from build123d import *

# Parameters (mm, degrees)
SKETCH1_R               = 3.3147
BOSS_EXTRUDE1_DEPTH     = 22.225
SHELL1_START            = -19.05
SHELL1_OUTLINE_R        = 3.3147
SHELL1_DEPTH            = 38.1
F_1_2_CLEARANCE_HOLE1_D = 13.49248


# Read off the part's stored shape, not the designer's step: Shell1
with BuildPart() as part:
    # Sketch1 → Boss-Extrude1 (new, symmetric)
    with BuildSketch(Plane.XY):
        Polygon((41.275, -44.45), (1101.725, -44.45), (1101.725, 0), (0, 0), (0, -3.175), align=None)
        with Locations((1076.325, -22.225)):
            Circle(SKETCH1_R, mode=Mode.SUBTRACT)
    extrude(amount=BOSS_EXTRUDE1_DEPTH, both=True)

    # Shell1 outline → Shell1 (cut)
    with BuildSketch(Plane.XY.offset(SHELL1_START)):
        Polygon((38.1, -41.275), (1101.725, -41.275), (1101.725, -3.175), (0, -3.175), align=None)
        with Locations((1076.325, -22.225)):
            Circle(SHELL1_OUTLINE_R, mode=Mode.SUBTRACT)
    extrude(amount=SHELL1_DEPTH, mode=Mode.SUBTRACT)

    # 1/2 Clearance Hole1 (through all)
    with Locations(Plane(origin=(0, 0, 0), x_dir=(1, 0, 0), z_dir=(0, 1, 0))):
        with Locations((19.05, 0)):
            Hole(F_1_2_CLEARANCE_HOLE1_D / 2)


solid = part.part
Here's how the part is built. I have some questions about the finished solid (model axes, mm). A direction names the side the tool comes from. Round coordinates to 2 decimals unless told otherwise and drop trailing zeros. Order: outer loops, then holes, each group sorted by start corner. A loop starts at its lowest first (then second) coordinate and runs counter-clockwise, first axis right, second up. Notation, with made-up numbers: M 22.5,-9.5 L 44.5,-9.5 A28 ccw 44.5,14.5 Z; hole C 36,-18 d3. An arc over 180 degrees is marked long. One line per question, with ' | ' between items.
1) Imagine slicing it at C-C, the plane y = -11.5. Write out the boundary of the cut face in (x, z) (3 decimals).
Checked values:
outline: M 8.325,-22.225 L 1101.725,-22.225 L 1101.725,-19.05 L 8.325,-19.05 Z; M 8.325,19.05 L 1101.725,19.05 L 1101.725,22.225 L 8.325,22.225 Z
2) On a 3-axis mill with a long thin cutter (end or side, diameter ignored), from which of +Z, -Z, +X, -X, +Y, -Y can I reach the whole of each face in a straight line? I mean faces 5 (the flat face through (562, -41.275, 0)), 6 (the flat face through (543, -22, -22.225)). Say none if no direction works.
Checked values:
face 5: +X, -X | face 6: -Z, +X, -X, +Y, -Y
3) Imagine slicing it at A-A, the plane x = 894.5. Write out the boundary of the cut face in (y, z) (3 decimals).
Checked values:
outline: M -44.45,-22.225 L 0,-22.225 L 0,22.225 L -44.45,22.225 Z; hole M -41.275,-19.05 L -3.175,-19.05 L -3.175,19.05 L -41.275,19.05 Z
4) I need wall thicknesses on line 1 (Z direction, x = 740.5, y = -11.5) (3 decimals); line 2 (Y direction, x = 676, z = -10) (3 decimals); line 3 (Z direction, x = 19, y = -1) (3 decimals). Which ranges of each line are inside material? Lowest first, please.
Checked values:
line 1: z = -22.225 to -19.05, 19.05 to 22.225 | line 2: y = -44.45 to -41.275, -3.175 to 0 | line 3: z = -22.225 to -6.746, 6.746 to 22.225
5) Imagine slicing it at B-B, the plane z = 0. Write out the boundary of the cut face in (x, y) (3 decimals), plus the area to 3 significant figures.
Checked values:
outline: M 0,-3.175 L 12.304,-3.175 L 12.304,0 L 0,0 Z; M 25.796,-3.175 L 1101.725,-3.175 L 1101.725,0 L 25.796,0 Z; M 38.1,-41.275 L 41.275,-44.45 L 1101.725,-44.45 L 1101.725,-41.275 Z | area: 6,830 mm²
6) We'd pull the mould along Z, two halves only. Please class faces 1 (the flat face through (543, -22, 22.225)), 2 (the flat face through (564, -44.45, 0)), 3 (the flat face through (543, -22, -19.05)), 4 (the flat face through (543, -22, 19.05)): released by +Z, released by -Z, zero draft, split by the parting line, or undercut.
Checked values:
face 1: released by +Z | face 2: zero draft | face 3: undercut | face 4: undercut
